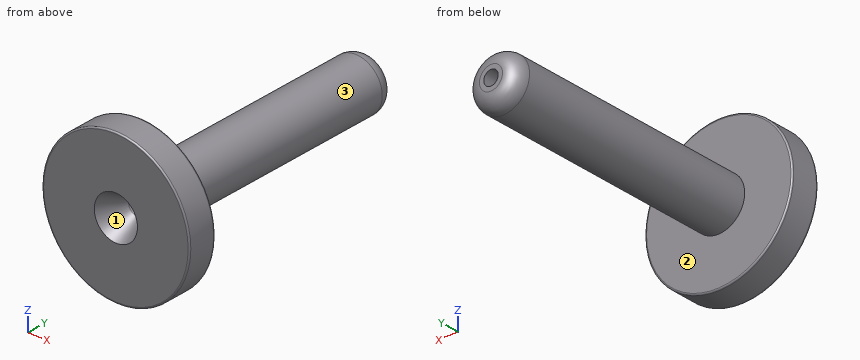
```python
from build123d import *

# Parameters (mm, degrees)
FILLET1_R = 6.35
FILLET2_R = 0.635
FILLET3_R = 2.54


with BuildPart() as part:
    # Sketch3 → Revolve1 (revolve)
    with BuildSketch(Plane.XY, mode=Mode.PRIVATE) as revolve1_sk:
        Polygon((3.175, 127), (3.175, 10.998522628), (9.525, 0), (32.500000024, 0), (32.500000024, 12.7), (11.43, 12.7), (11.43, 127), align=None)
    revolve(revolve1_sk.sketch.rotate(Axis((0, 0, 0), (0, 1, 0)), 90), axis=Axis((0, 0, 0), (0, 1, 0)))

    # Fillet1
    fillet1_edges = [part.edges().sort_by_distance(p)[0] for p in [
        (0, 127, 11.43),
    ]]
    fillet(fillet1_edges, radius=FILLET1_R)

    # Fillet2
    fillet2_edges = [part.edges().sort_by_distance(p)[0] for p in [
        (0, 12.7, 32.500000024),
        (0, 0, 32.500000024),
    ]]
    fillet(fillet2_edges, radius=FILLET2_R)

    # Fillet3
    fillet3_edges = [part.edges().sort_by_distance(p)[0] for p in [
        (0, 10.998522628, 3.175),
    ]]
    fillet(fillet3_edges, radius=FILLET3_R)


solid = part.part
```
The model under review builds one solid part; all positions refer to its coordinate system, in mm. Face numbers are marked on the shaded views. Round coordinates to 2 decimals unless told otherwise and drop trailing zeros. Write each loop counter-clockwise with the first axis right and the second up, starting at its lowest first coordinate (ties: lowest second). Pieces come first, ordered by that corner, then holes. Notation, with made-up numbers: (87.25, 49.25) - (103.25, 49.25) arc R12 cw to (103.25, 66.25) - close; hole circle Ø10 at (76, 8). An arc over 180 degrees is marked (long way). One line per question, with ' | ' between items.
Item 1: For P1, Ø8, axis at x = 24.5, z = -18.5, coming from the +Y side; P2, Ø8.5, axis at x = 0, z = 0, coming from the +Y side; P3, Ø5, axis at y = 102, z = -14, coming from the +X side; P4, Ø5, axis at x = -8.5, y = 108.5, coming from the -Z side, all flat-tipped, find the tip position at first contact; note any pin that passes through.
Resolved:
P1: stops at y = 12.7 | P2: stops at y = 127 | P3: passes through | P4: stops at z = -9.73
Item 2: Add section A-A, the plane y = 37. Give the boundary of the cut face in (x, z) (3 decimals).
Resolved:
outline: circle Ø22.86 at (0, 0); hole circle Ø6.35 at (0, 0)
Item 3: The part is to be moulded in two halves that separate along Z. For the marked faces 1, 2 and 3, say which applies: pulls with the +Z half, pulls with the -Z half, needs draft (parallel to the pull), parting line crosses it, or undercut.
Resolved:
face 1: undercut | face 2: needs draft | face 3: parting line crosses it
Item 4: To check wall thickness, follow probe 1 along X at (y, z) = (74, 0) (3 decimals); probe 2 along Y at (x, z) = (7.5, 24.5); probe 3 along X at (y, z) = (85, 2). State the ranges of each line that lie inside material, in increasing order.
Resolved:
probe 1: x = -11.43 to -3.175, 3.175 to 11.43 | probe 2: y = 0 to 12.7 | probe 3: x = -11.25 to -2.47, 2.47 to 11.25
